The listing builds one solid part. Answer for the finished solid, in the listing's coordinates (mm). A direction names the side the tool comes from. Give positions to 0.01 mm unless a question says otherwise; leave off trailing zeros. Order: outer loops, then holes, each group sorted by start corner. A loop starts at its lowest first (then second) coordinate and runs counter-clockwise, first axis right, second up. Notation, with made-up numbers: (-12.75, 85) -> (2.25, 85) arc R33 cw to (2.25, 113) -> close; hole circle Ø3 at (63.5, 84.25). An arc over 180 degrees is marked (long way). Answer as a JSON object with one key per item and string values. Group by question number.
```python
from build123d import *

# Parameters (mm, degrees)
SKETCH1_W           = 6.5
SKETCH1_H           = 92.5
BOSS_EXTRUDE1_DEPTH = 10
SKETCH2_W           = 3.25
SKETCH2_H           = 90
CUT_EXTRUDE1_DEPTH  = 10
CHAMFER1_SIZE       = 2
BOSS_EXTRUDE2_DEPTH = 3.25
SKETCH6_W           = 2.05
SKETCH6_H           = 8.8
CUT_EXTRUDE2_DEPTH  = 80


with BuildPart() as part:
    # Sketch1 → Boss-Extrude1 (new body)
    with BuildSketch(Plane.XY):
        Rectangle(SKETCH1_W, SKETCH1_H)
    extrude(amount=BOSS_EXTRUDE1_DEPTH)

    # Sketch2 → Cut-Extrude1 (cut)
    with BuildSketch(Plane.XY.offset(10)):
        with Locations((-1.625, 1.25)):
            Rectangle(SKETCH2_W, SKETCH2_H)
    extrude(amount=-CUT_EXTRUDE1_DEPTH, mode=Mode.SUBTRACT)

    # Chamfer1
    chamfer1_edges = [part.edges().sort_by_distance(p)[0] for p in [
        (-3.25, -46.25, 5),
    ]]
    chamfer(chamfer1_edges, length=CHAMFER1_SIZE)

    # Sketch4 → Boss-Extrude2 (add)
    with BuildSketch(Plane.ZY):
        Polygon((10, -8.75), (11, -8.75), (11, -6.85), (10.55, -6.85), (10.55, -7.85), (10, -7.85), align=None)
    boss_extrude2 = extrude(amount=-BOSS_EXTRUDE2_DEPTH)

    # Mirror1: Boss-Extrude2 across plane
    add(boss_extrude2.mirror(Plane.XY.offset(5)))

    # Sketch6 → Cut-Extrude2 (cut)
    with BuildSketch(Plane(origin=(0, 46.25, 0), x_dir=(1, 0, 0), z_dir=(0, 1, 0))):
        with Locations((1.625, -5)):
            Rectangle(SKETCH6_W, SKETCH6_H)
    extrude(amount=-CUT_EXTRUDE2_DEPTH, mode=Mode.SUBTRACT)


solid = part.part
```
(1) Which of the six approach directions +Z, -Z, +X, -X, +Y, -Y give full straight-line access (tool end or side, diameter ignored) to faces 4 (the flat face through (1, -46.25, 5)), 5 (the flat face through (1, -27, 0)), 6 (the flat face through (2, 7, 9.4)), 7 (the flat face through (1, -27, 10)), 8 (the flat face through (-2, -43.75, 5))?
(2) For a pull along X with two mould halves and no side action, classify faces 1 (the flat face through (2, 7, 0.6)), 2 (the flat face through (2, -8, -1)), 3 (the flat face through (-2.2, -45.3, 4.9)) as +X half, -X half, draft (parallel to the pull), parting line (faces both ways), or undercut.
(3) A cutting plane is placed at B-B (y = -24). Determine the outline of the cut face in (x, z), and give its area (3 significant figures).
(4) Flat-ended cylindrical pins translate along their axes: pin 1 Ø3.5 at (x, z) = (-2.5, 3.5) entering from +Y; pin 2 Ø0.6 at (x, y) = (1.5, 25.5) entering from +Z; pin 3 Ø3 at (x, z) = (1, 7) entering from +Y; pin 4 Ø0.6 at (x, y) = (1.5, 10.5) entering from -Z. Find the tip coordinate at first contact, or state that the pin passes through.
(5) A cutting plane is placed at D-D (x = -2.5). Determine the outline of the cut face in (y, z), and give its area (3 significant figures).
(6) Find the intervals of material crossed by line 1 along X through (y, z) = (-20.5, 7.75); line 2 along Z through (x, y) = (1.5, 14); line 3 along Z through (x, y) = (3, 23), in increasing order. Write a range as [from, to].
(7) A cutting plane is placed at C-C (x = 1.75). Determine the outline of the cut face in (y, z), and give its area (3 significant figures).
(8) A cutting plane is placed at A-A (z = 8.25). Determine the outline of the cut face in (x, y).
Check sheet entries:
{
 "1": {"face 4": "+Z, -Z, +X, -X, -Y", "face 5": "-Z, +X, -X, -Y", "face 6": "+Y", "face 7": "+Z, +X, -X, -Y", "face 8": "+Z, -Z, -X, +Y"},
 "2": {"face 1": "undercut", "face 2": "draft", "face 3": "-X half"},
 "3": {"outline": "(0, 0) -> (3.25, 0) -> (3.25, 10) -> (0, 10) -> close; hole (0.6, 0.6) -> (2.65, 0.6) -> (2.65, 9.4) -> (0.6, 9.4) -> close", "area": "14.5 mm2"},
 "4": {"pin 1": "stops at y = -43.75", "pin 2": "stops at z = 10", "pin 3": "stops at y = 46.25", "pin 4": "stops at z = 0"},
 "5": {"outline": "(-45, 0) -> (-43.75, 0) -> (-43.75, 10) -> (-45, 10) -> close", "area": "12.5 mm2"},
 "6": {"line 1": "x = [0, 0.6], [2.65, 3.25]", "line 2": "z = [0, 0.6], [9.4, 10]", "line 3": "z = [0, 10]"},
 "7": {"outline": "(-46.25, 0) -> (-8.75, 0) -> (-8.75, -1) -> (-6.85, -1) -> (-6.85, -0.55) -> (-7.85, -0.55) -> (-7.85, 0) -> (46.25, 0) -> (46.25, 0.6) -> (-33.75, 0.6) -> (-33.75, 9.4) -> (46.25, 9.4) -> (46.25, 10) -> (-7.85, 10) -> (-7.85, 10.55) -> (-6.85, 10.55) -> (-6.85, 11) -> (-8.75, 11) -> (-8.75, 10) -> (-46.25, 10) -> close", "area": "224 mm2"},
 "8": {"outline": "(-3.25, -44.25) -> (-1.25, -46.25) -> (3.25, -46.25) -> (3.25, 46.25) -> (2.65, 46.25) -> (2.65, -33.75) -> (0.6, -33.75) -> (0.6, 46.25) -> (0, 46.25) -> (0, -43.75) -> (-3.25, -43.75) -> close"}
}
